CAD build for the part. Positions are in the model's coordinates, mm. A direction names the side the tool comes from. Coordinates: 2 decimals unless noted, no trailing zeros. Loops run counter-clockwise (first coordinate to the right, second up) from the corner with the lowest first, then second, coordinate; pieces in that order, holes last. Notation, with made-up numbers: (76, 16) -> (124, 16) arc R16 ccw to (124, 29) -> close; hole circle Ø6 at (69.5, 88). An arc over 180 degrees is marked (long way). Answer as CSV lines item,"result". Start each with the question number.
from build123d import *

# Parameters (mm, degrees)
SKETCH1_W           = 150
SKETCH1_H           = 30
BOSS_EXTRUDE1_DEPTH = 5
SKETCH3_W           = 150
SKETCH3_H           = 5
BOSS_EXTRUDE2_DEPTH = 25
SKETCH6_R           = 7.5
SKETCH6_R_2         = 5
CUT_EXTRUDE2_DEPTH  = 25
SKETCH7_R           = 2.5
CUT_EXTRUDE3_DEPTH  = 25
CHAMFER1_SIZE       = 1
FILLET2_R           = 2
SKETCH8_W           = 43.274843737
SKETCH8_H           = 64.613346869
CUT_EXTRUDE4_DEPTH  = 120
FILLET3_R           = 2


with BuildPart() as part:
    # Sketch1 → Boss-Extrude1 (new body)
    with BuildSketch(Plane(origin=(0, 0, 0), x_dir=(1, 0, 0), z_dir=(0, 1, 0))):
        with Locations((22.308802864, -0.815715524)):
            Rectangle(SKETCH1_W, SKETCH1_H)
    extrude(amount=BOSS_EXTRUDE1_DEPTH)

    # Sketch3 → Boss-Extrude2 (add)
    with BuildSketch(Plane(origin=(0, 5, 0), x_dir=(1, 0, 0), z_dir=(0, 1, 0))):
        with Locations((22.308802864, 11.684284476)):
            Rectangle(SKETCH3_W, SKETCH3_H)
    extrude(amount=BOSS_EXTRUDE2_DEPTH)

    # Sketch6 → Cut-Extrude2 (cut)
    with BuildSketch(Plane(origin=(0, 5, 0), x_dir=(1, 0, 0), z_dir=(0, 1, 0))):
        with Locations(Location((82.308802864, -0.815715524, 0), (0, 0, 90))):
            Circle(SKETCH6_R)
        with Locations(Location((54.808802864, -8.315715524, 0), (0, 0, 90))):
            Circle(SKETCH6_R_2)
        with Locations(Location((29.808802864, -8.315715524, 0), (0, 0, 90))):
            Circle(SKETCH6_R_2)
        with Locations(Location((2.308802864, -8.315715524, 0), (0, 0, 90))):
            Circle(SKETCH6_R_2)
        with Locations(Location((-37.691197136, -8.315715524, 0), (0, 0, 90))):
            Circle(SKETCH6_R_2)
    extrude(amount=-CUT_EXTRUDE2_DEPTH, mode=Mode.SUBTRACT)

    # Sketch7 → Cut-Extrude3 (cut)
    with BuildSketch(Plane.XY.offset(-9.184284476)):
        with Locations((82.308802864, 17.478664245)):
            Circle(SKETCH7_R)
        with Locations((-37.691197136, 17.478664245)):
            Circle(SKETCH7_R)
        with Locations((22.308802864, 17.478664245)):
            Circle(SKETCH7_R)
    extrude(amount=-CUT_EXTRUDE3_DEPTH, mode=Mode.SUBTRACT)

    # Chamfer1
    chamfer1_edges = [part.edges().sort_by_distance(p)[0] for p in [
        (79.808802864, 17.478664245, -9.184284476),
        (-40.191197136, 17.478664245, -9.184284476),
        (19.808802864, 17.478664245, -9.184284476),
    ]]
    chamfer(chamfer1_edges, length=CHAMFER1_SIZE)

    # Fillet2
    fillet2_edges = [part.edges().sort_by_distance(p)[0] for p in [
        (22.308802864, 5, 15.815715524),
        (22.308802864, 0, 15.815715524),
        (22.308802864, 5, -9.184284476),
        (-52.691197136, 30, -11.684284476),
        (97.308802864, 30, -11.684284476),
    ]]
    fillet(fillet2_edges, radius=FILLET2_R)

    # Sketch8 → Cut-Extrude4 (cut)
    with BuildSketch(Plane.ZY.offset(52.691197136)):
        with Locations((-0.153926337, 8.461505149)):
            Rectangle(SKETCH8_W, SKETCH8_H)
    extrude(amount=-CUT_EXTRUDE4_DEPTH, mode=Mode.SUBTRACT)

    # Fillet3
    fillet3_edges = [part.edges().sort_by_distance(p)[0] for p in [
        (67.308802864, 30, -11.684284476),
    ]]
    fillet(fillet3_edges, radius=FILLET3_R)


solid = part.part
Item 1: Saw through at B-B (x = 93). Write the cut outline in (y, z), plus the area to 3 significant figures.
Item 2: Flat gauge pins, fed straight in: pin 1 Ø1.5 at (x, y) = (90.5, 27) entering from +Z; pin 2 Ø10.5 at (x, z) = (82, -1.5) entering from +Y; pin 3 Ø2 at (x, z) = (88, -4.5) entering from -Y. Where does each tip first touch, or does it go through?
Item 3: Which spindle directions (+Z, -Z, +X, -X, +Y, -Y) get a long thin tool onto all of the face, cutting with end or side? Do faces 1 (the face through (79, 5, 8)), 2 (the face through (97.309, 4, -5)). Say none if no direction does.
Item 4: Wall check: probe 1 along Z at (x, y) = (95.5, 16.75); probe 2 along Y at (x, z) = (84, -10.75); probe 3 along Y at (x, z) = (91.25, -2.5). Give the ranges that are in metal, low to high.
Item 5: Two-plate mould, pull along Y, no slides. Class faces 3 (the face through (82.519, 4.43, 15.214)), 4 (the face through (85, 0, -7)), 5 (the face through (84.693, 18.23, -12.156)), 6 (the face through (82.1, 14.8, -14.184)): pulls with the +Y half, pulls with the -Y half, needs draft (parallel to the pull), parting line crosses it, or undercut.
Item 6: Saw through at D-D (y = 2.5). Write the cut outline in (x, z).
Item 7: Saw through at C-C (x = 75.25). Write the cut outline in (y, z), plus the area to 3 significant figures.
Item 8: Saw through at A-A (z = 2). Write the cut outline in (x, y), plus the area to 3 significant figures.
Geometry check:
1,outline,"(0, -14.18) -> (30, -14.18) -> (30, -9.18) -> (7, -9.18) arc R2 cw to (5, -7.18) -> (5, 13.82) arc R2 ccw to (3, 15.82) -> (2, 15.82) arc R2 ccw to (0, 13.82) -> close"
1,area,"274 mm2"
2,pin 1,"z = -9.18"
2,pin 2,"y = 5"
2,pin 3,"y = 0"
3,face 1,"+Z, +X, -X, +Y"
3,face 2,"+Z, -Z, +X, +Y, -Y"
4,probe 1,"-14.18 to -9.18"
4,probe 2,"0 to 15.64, 19.32 to 30"
4,probe 3,"0 to 5"
5,face 3,"pulls with the +Y half"
5,face 4,"pulls with the -Y half"
5,face 5,"undercut"
5,face 6,"needs draft"
6,outline,"(67.31, -14.18) -> (97.31, -14.18) -> (97.31, 15.82) -> (67.31, 15.82) -> close; hole circle Ø15 at (82.31, 0.82)"
7,outline,"(0, -14.18) -> (30, -14.18) -> (30, -9.18) -> (7, -9.18) arc R2 cw to (5, -7.18) -> (5, -1.72) -> (0, -1.72) -> close; (0, 3.35) -> (5, 3.35) -> (5, 13.82) arc R2 ccw to (3, 15.82) -> (2, 15.82) arc R2 ccw to (0, 13.82) -> close"
7,area,"249 mm2"
8,outline,"(67.31, 0) -> (74.9, 0) -> (74.9, 5) -> (67.31, 5) -> close; (89.71, 0) -> (97.31, 0) -> (97.31, 5) -> (89.71, 5) -> close"
8,area,"75.9 mm2"
